```python
from build123d import *

# Parameters (mm, degrees)
MODEL_R             = 3.6
MODEL_R_2           = 2.5
BOSS_EXTRUDE1_DEPTH = 3


with BuildPart() as part:
    # Model → Boss-Extrude1 (new body)
    with BuildSketch(Plane.XY):
        with BuildLine():
            Line((-75.3, 0), (75.3, 0))
            ThreePointArc((75.3, 0), (87.8, 12.5), (75.3, 25))
            Line((75.3, 25), (45.873401872, 25))
            ThreePointArc((45.873401872, 25), (44.974095806, 25.178883099), (44.211700936, 25.688299064))
            Line((44.211700936, 25.688299064), (25.688299064, 44.211700936))
            ThreePointArc((25.688299064, 44.211700936), (25.178883099, 44.974095805), (25, 45.873401872))
            Line((25, 45.873401872), (25, 78.926598129))
            ThreePointArc((25, 78.926598129), (25.178883099, 79.825904195), (25.688299064, 80.588299064))
            Line((25.688299064, 80.588299064), (44.211700936, 99.111700936))
            ThreePointArc((44.211700936, 99.111700936), (44.974095806, 99.621116901), (45.873401872, 99.8))
            Line((45.873401872, 99.8), (75.3, 99.8))
            ThreePointArc((75.3, 99.8), (87.8, 112.3), (75.3, 124.8))
            Line((75.3, 124.8), (25.973401872, 124.8))
            ThreePointArc((25.973401872, 124.8), (25.074095806, 124.621116901), (24.311700936, 124.111700936))
            Line((24.311700936, 124.111700936), (5.688299064, 105.488299064))
            ThreePointArc((5.688299064, 105.488299064), (4.925904195, 104.978883099), (4.026598129, 104.8))
            Line((4.026598129, 104.8), (-4.026598129, 104.8))
            ThreePointArc((-4.026598129, 104.8), (-4.925904195, 104.978883099), (-5.688299064, 105.488299064))
            Line((-5.688299064, 105.488299064), (-24.311700936, 124.111700936))
            ThreePointArc((-24.311700936, 124.111700936), (-25.074095806, 124.621116901), (-25.973401872, 124.8))
            Line((-25.973401872, 124.8), (-75.3, 124.8))
            ThreePointArc((-75.3, 124.8), (-87.8, 112.3), (-75.3, 99.8))
            Line((-75.3, 99.8), (-45.873401872, 99.8))
            ThreePointArc((-45.873401872, 99.8), (-44.974095806, 99.621116901), (-44.211700936, 99.111700936))
            Line((-44.211700936, 99.111700936), (-25.688299064, 80.588299064))
            ThreePointArc((-25.688299064, 80.588299064), (-25.178883099, 79.825904195), (-25, 78.926598129))
            Line((-25, 78.926598129), (-25, 45.873401872))
            ThreePointArc((-25, 45.873401872), (-25.178883099, 44.974095805), (-25.688299064, 44.211700936))
            Line((-25.688299064, 44.211700936), (-44.211700936, 25.688299064))
            ThreePointArc((-44.211700936, 25.688299064), (-44.974095806, 25.178883099), (-45.873401872, 25))
            Line((-45.873401872, 25), (-75.3, 25))
            ThreePointArc((-75.3, 25), (-87.8, 12.5), (-75.3, 0))
        make_face()
        with Locations((75.3, 12.5)):
            Circle(MODEL_R, mode=Mode.SUBTRACT)
        with Locations((0, 12.5)):
            Circle(MODEL_R, mode=Mode.SUBTRACT)
        with Locations((-75.3, 12.5)):
            Circle(MODEL_R, mode=Mode.SUBTRACT)
        with Locations((-35.3, 112.3)):
            Circle(MODEL_R_2, mode=Mode.SUBTRACT)
        with Locations((-75.3, 112.3)):
            Circle(MODEL_R_2, mode=Mode.SUBTRACT)
        with Locations((35.3, 112.3)):
            Circle(MODEL_R_2, mode=Mode.SUBTRACT)
        with Locations((75.3, 112.3)):
            Circle(MODEL_R_2, mode=Mode.SUBTRACT)
        with BuildLine():
            Line((26.57, 99.43), (26.57, 108.43))
            ThreePointArc((26.57, 108.43), (23.57, 111.43), (20.57, 108.43))
            Line((20.57, 108.43), (20.57, 99.43))
            ThreePointArc((20.57, 99.43), (23.57, 96.43), (26.57, 99.43))
        make_face(mode=Mode.SUBTRACT)
        with BuildLine():
            Line((-26.57, 99.43), (-26.57, 108.43))
            ThreePointArc((-26.57, 108.43), (-23.57, 111.43), (-20.57, 108.43))
            Line((-20.57, 108.43), (-20.57, 99.43))
            ThreePointArc((-20.57, 99.43), (-23.57, 96.43), (-26.57, 99.43))
        make_face(mode=Mode.SUBTRACT)
    extrude(amount=BOSS_EXTRUDE1_DEPTH)


solid = part.part
```
Can you work these out from the model? Positions are in its coordinate system, mm. A direction names the side the tool comes from. Coordinates: 2 decimals unless noted, no trailing zeros. Loops run counter-clockwise (first coordinate to the right, second up) from the corner with the lowest first, then second, coordinate; pieces in that order, holes last. Notation, with made-up numbers: (7, -33.5) - (31, -33.5) arc R10 cw to (31, -20.5) - close; hole circle Ø1 at (-39.75, 23). An arc over 180 degrees is marked (long way). Answer as CSV lines item,"result". Start each with the question number.
1) Suppose I cut it at B-B (x = 49). Please give me the cut outline in (y, z).
2) Suppose I cut it at A-A (y = 12.5). Please give me the cut outline in (x, z).
3) Suppose I cut it at C-C (x = 0). Please give me the cut outline in (y, z), plus the area to 3 significant figures.
4) Suppose I cut it at D-D (z = 0.9). Count the separate pieces of the cut face and the enclosed holes in it, plus the area to 3 significant figures.
5) Which directions (+Z, -Z, +X, -X, +Y, -Y) give clear straight access to the entire face, cutting with the end or side of a thin tool? Please do faces 1 (the flat face through (-35.1, 90, 1.5)), 2 (the flat face through (34.8, 89.7, 1.5)), 3 (the cylindrical face through (74.76, 109.86, 1.48)), 4 (the flat face through (-14.9, 114.7, 1.5)).
6) I need wall thicknesses on line 1 (Y direction, x = -75.3, z = 2); line 2 (X direction, y = 109, z = 1.7); line 3 (X direction, y = 102.5, z = 2.6). Which ranges of each line are inside material? Lowest first, please. Write a range as from..to.
7) For pin 1 (1.5 mm diameter, centred on x = 66, z = 2, fed in from -Y); pin 2 (1.5 mm diameter, centred on y = 105.5, z = 2, fed in from +X); pin 3 (0.9 mm diameter, centred on y = 67.5, z = 1.5, fed in from -X); pin 4 (4.5 mm diameter, centred on x = -75.3, y = 112.3, fed in from +Z), each with a flat end and sliding along its axis, tell me the tip position at first contact or that it passes through.
8) Thinking about a two-plate mould opening in Y: for faces 5 (the flat face through (15.1, 114.9, 1.5)), 6 (the flat face through (35.1, 34.8, 1.5)), 7 (the flat face through (-1, 63, 3)), which applies, pulls with the +Y half, pulls with the -Y half, needs draft (parallel to the pull), parting line crosses it, or undercut?
Check result:
1,outline,"(0, 0) - (25, 0) - (25, 3) - (0, 3) - close; (99.8, 0) - (124.8, 0) - (124.8, 3) - (99.8, 3) - close"
2,outline,"(-87.8, 0) - (-78.9, 0) - (-78.9, 3) - (-87.8, 3) - close; (-71.7, 0) - (-3.6, 0) - (-3.6, 3) - (-71.7, 3) - close; (3.6, 0) - (71.7, 0) - (71.7, 3) - (3.6, 3) - close; (78.9, 0) - (87.8, 0) - (87.8, 3) - (78.9, 3) - close"
3,outline,"(0, 0) - (8.9, 0) - (8.9, 3) - (0, 3) - close; (16.1, 0) - (104.8, 0) - (104.8, 3) - (16.1, 3) - close"
3,area,"293 mm²"
4,separate pieces,"1"
4,enclosed holes,"9"
4,area,"12,100 mm²"
5,face 1,"+Z, -Z, -X"
5,face 2,"+Z, -Z, +X"
5,face 3,"+Z, -Z"
5,face 4,"+Z, -Z, +Y"
6,line 1,"y = 0..8.9, 16.1..25, 99.8..109.8, 114.8..124.8"
6,line 2,"x = -87.36..-26.52, -20.62..-9.2, 9.2..20.62, 26.52..87.36"
6,line 3,"x = -83.06..-26.57, -20.57..20.57, 26.57..83.06"
7,pin 1,"stops at y = 0"
7,pin 2,"stops at x = 86.24"
7,pin 3,"stops at x = -25"
7,pin 4,"passes through"
8,face 5,"pulls with the +Y half"
8,face 6,"undercut"
8,face 7,"needs draft"
